```python
from build123d import *

# Parameters (mm, degrees)
SKETCH2_W           = 152.4
SKETCH2_H           = 101.6
BOSS_EXTRUDE1_DEPTH = 50.8
SKETCH3_W           = 50.8
SKETCH3_H           = 76.2
CUT_EXTRUDE1_DEPTH  = 137.783186101
SKETCH4_W           = 25.4
SKETCH4_H           = 25.4
CUT_EXTRUDE2_DEPTH  = 120.1365603
SKETCH5_W           = 25.4
SKETCH5_H           = 50.8
CUT_EXTRUDE3_DEPTH  = 76.2
SKETCH6_W           = 25.4
SKETCH6_H           = 25.4
CUT_EXTRUDE4_DEPTH  = 137.783186101
CHAMFER1_SIZE2      = 101.6
CHAMFER1_SIZE       = 50.8
SKETCH7_RX          = 25.4
SKETCH7_RY          = 12.7
CUT_EXTRUDE5_DEPTH  = 120.1365603


with BuildPart() as part:
    # Sketch2 → Boss-Extrude1 (new, symmetric)
    with BuildSketch(Plane.XY):
        Rectangle(SKETCH2_W, SKETCH2_H)
    extrude(amount=BOSS_EXTRUDE1_DEPTH, both=True)

    # Sketch3 → Cut-Extrude1 (cut, through all)
    with BuildSketch(Plane.XY.offset(50.8)):
        with Locations((50.8, 12.7)):
            Rectangle(SKETCH3_W, SKETCH3_H)
    extrude(amount=-CUT_EXTRUDE1_DEPTH, mode=Mode.SUBTRACT)

    # Sketch4 → Cut-Extrude2 (cut, through all)
    with BuildSketch(Plane(origin=(0, -25.4, 0), x_dir=(1, 0, 0), z_dir=(0, 1, 0))):
        with Locations((63.5, -38.1)):
            Rectangle(SKETCH4_W, SKETCH4_H)
    extrude(amount=-CUT_EXTRUDE2_DEPTH, mode=Mode.SUBTRACT)

    # Sketch5 → Cut-Extrude3 (cut)
    with BuildSketch(Plane(origin=(0, 50.8, 0), x_dir=(1, 0, 0), z_dir=(0, 1, 0))):
        with Locations((12.7, -25.4)):
            Rectangle(SKETCH5_W, SKETCH5_H)
    extrude(amount=-CUT_EXTRUDE3_DEPTH, mode=Mode.SUBTRACT)

    # Sketch6 → Cut-Extrude4 (cut, through all)
    with BuildSketch(Plane(origin=(0, 0, -50.8), x_dir=(-1, 0, 0), z_dir=(0, 0, -1))):
        with Locations((63.5, 38.1)):
            Rectangle(SKETCH6_W, SKETCH6_H)
    extrude(amount=-CUT_EXTRUDE4_DEPTH, mode=Mode.SUBTRACT)

    # Chamfer1
    chamfer1_edges = [part.edges().sort_by_distance(p)[0] for p in [
        (-25.4, 50.8, 50.8),
    ]]
    chamfer1_side = [part.faces().sort_by_distance(p)[0] for p in [
        (-25.4, 49.784, 50.8),
    ]]
    chamfer(chamfer1_edges, length=CHAMFER1_SIZE - 0.0001, length2=CHAMFER1_SIZE2 - 0.0001, reference=chamfer1_side[0])  # a hair under: the kernel refuses the full size

    # Sketch7 → Cut-Extrude5 (cut, through all)
    with BuildSketch(Plane(origin=(0, -25.4, 0), x_dir=(1, 0, 0), z_dir=(0, 1, 0))):
        with Locations(Location((50.8, 12.7), (0, 0, -90))):
            Ellipse(SKETCH7_RX, SKETCH7_RY)
    extrude(amount=-CUT_EXTRUDE5_DEPTH, mode=Mode.SUBTRACT)


solid = part.part
```
Design review of the part built by this model. Coordinates are the model's own, in mm. A direction names the side the tool comes from. Coordinates: 2 decimals unless noted, no trailing zeros. Order: outer loops, then holes, each group sorted by start corner. A loop starts at its lowest first (then second) coordinate and runs counter-clockwise, first axis right, second up.
1) Take a section at B-B, the plane y = -18.5. Give the boundary of the cut face in (x, z), and give its area (3 significant figures).
2) Take a section at C-C, the plane z = 14.5. Give the boundary of the cut face in (x, y), and give its area (3 significant figures).
3) Wall thickness on line 1 along X through (y, z) = (-26, -12.5); line 2 along Y through (x, z) = (32, 17); line 3 along X through (y, z) = (-10.5, 15): over which ranges is each line inside the solid? List them lowest first.
4) Clearance check with flat-ended pins moving along their axes: pin 1 (5 mm diameter, centred on x = 9, z = 38.5, fed in from +Y); pin 2 (20.5 mm diameter, centred on x = -63, z = -35.5, fed in from +Y); pin 3 (20.5 mm diameter, centred on y = 32, z = -32, fed in from -X); pin 4 (2 mm diameter, centred on y = 8.5, z = 14.5, fed in from +X). State where each tip first meets the part, or that it passes through.
5) For faces 1 (the flat face through (25.4, 4, -25)), 2 (the flat face through (-18, -11, -50.8)), 3 (the flat face through (-63, 25.4, -26)), 4 (the flat face through (50.8, -38, 38)), 5 (the flat face through (38, -25.4, 1)), list the 3-axis set-ups (+Z, -Z, +X, -X, +Y, -Y) from which the entire face can be reached by the end or side of a thin tool; tool diameter is ignored.
Returned:
1. outline: (-76.2, -50.8) - (25.4, -50.8) - (25.4, 0) - (0, 0) - (0, 50.8) - (-76.2, 50.8) - close
1. area: 9,030 mm2
2. outline: (-76.2, -50.8) - (76.2, -50.8) - (76.2, -25.4) - (0, -25.4) - (0, 18.15) - (-76.2, 18.15) - close
2. area: 7,190 mm2
3. line 1: x = -76.2 to 38.1, 63.5 to 76.2
3. line 2: y = -50.8 to -25.4
3. line 3: x = -76.2 to 0
4. pin 1: stops at y = -25.4
4. pin 2: stops at y = 25.4
4. pin 3: stops at x = -76.2
4. pin 4: stops at x = 0
5. face 1: +Z, -Z, +X, +Y
5. face 2: -Z, +X, -X, +Y, -Y
5. face 3: +Z, -Z, -X, +Y
5. face 4: +Z, +X, +Y, -Y
5. face 5: +Z, +X, +Y
